Input: part model. Units: mm. Frame: model coordinates. Face numbers are marked on the shaded views. A direction names the side the tool comes from. Round coordinates to 2 decimals unless told otherwise and drop trailing zeros. Loops run counter-clockwise (first coordinate to the right, second up) from the corner with the lowest first, then second, coordinate; pieces in that order, holes last. Notation, with made-up numbers: (-38.75, 2.25) - (-1.75, 2.25) arc R24 ccw to (-1.75, 18.25) - close; hole circle Ø2 at (-16, 70.25). An arc over 180 degrees is marked (long way). Write each question's results on one line, items separated by ' | '.
from build123d import *

# Parameters (mm, degrees)
F0_R     = 4.1
F0_R_2   = 1.625
F1_DEPTH = 15


with BuildPart() as f1:
    # F0 (on Top) → F1 (new body)
    with BuildSketch(Plane.XY):
        with BuildLine():
            Line((19.449329, 20.047105), (-17.462153, 20.047105))
            ThreePointArc((-17.462153, 20.047105), (-21.400342, 15.5), (-17.462153, 10.952895))
            ThreePointArc((-17.462153, 10.952895), (-13.583628, 11.018037), (-9.926019, 12.30997))
            ThreePointArc((-9.926019, 12.30997), (-0.583426, 14.431472), (8.979468, 13.851907))
            ThreePointArc((8.979468, 13.851907), (9.394135, 9.361936), (8.242019, 5.002531))
            ThreePointArc((8.242019, 5.002531), (7.672541, 2.530704), (7.5, 0))
            ThreePointArc((7.5, 0), (9.673183, -5.326817), (15, -7.5))
            ThreePointArc((15, -7.5), (20.326817, -5.326817), (22.5, 0))
            ThreePointArc((22.5, 0), (22.327459, 2.530704), (21.757981, 5.002531))
            ThreePointArc((21.757981, 5.002531), (21.215093, 9.858766), (22.510411, 14.570442))
            ThreePointArc((22.510411, 14.570442), (22.434346, 18.121727), (19.449329, 20.047105))
        make_face()
        with Locations((15, 0)):
            Circle(F0_R, mode=Mode.SUBTRACT)
        with Locations((15.5, 15.5)):
            Circle(F0_R_2, mode=Mode.SUBTRACT)
    extrude(amount=F1_DEPTH)


solid = f1.part
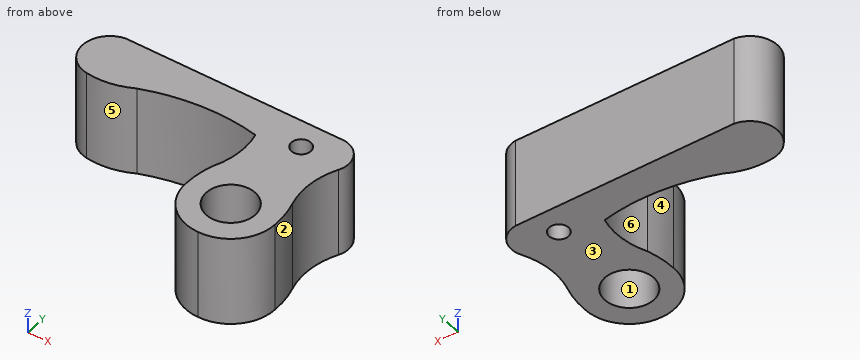
1. Line query: line 1 (Y direction, x = 15.5, z = 9) (3 decimals); line 2 (Y direction, x = 15, z = 12); line 3 (X direction, y = 15.75, z = 7.75). Output: solid intervals per line, ascending. Write a range as [from, to].
Answer:
line 1: [-7.488, -4.069], [4.069, 13.875], [17.125, 20.047] | line 2: [-7.5, -4.1], [4.1, 13.95], [17.05, 20.05] | line 3: [-21.39, 13.89], [17.11, 22.88]
2. Set-up query: the marked faces 1 and 2. Return all of +Z, -Z, +X, -X, +Y, -Y with unobstructed straight access to the full face (end or side cutting, diameter ignored); none if empty.
Answer:
face 1: +Z, -Z | face 2: +Z, -Z, +X
3. Section query D-D, the plane y = 15.5. Output: boundary loops of the cut face in (x, z) (1 decimal).
Answer:
outline: (-21.4, 0) - (13.9, 0) - (13.9, 15) - (-21.4, 15) - close; (17.1, 0) - (22.8, 0) - (22.8, 15) - (17.1, 15) - close
4. Contact query for flat-ended pins moving along their axis: pin 1 (3 mm diameter, centred on x = 12.5, z = 8, fed in from -Y); pin 2 (5 mm diameter, centred on y = 12.5, z = 11.5, fed in from +X); pin 3 (4 mm diameter, centred on x = 5, z = 6.5, fed in from -Y); pin 4 (13 mm diameter, centred on x = 15, y = 0, fed in from -Z). Output: stop coordinate, or through.
Answer:
pin 1: y = -7.44 | pin 2: x = 22.69 | pin 3: y = 14.2 | pin 4: z = 0
5. Section query B-B, the plane z = 14.25. Output: boundary loops of the cut face in (x, y) (3 decimals), plus the area to 3 significant figures.
Answer:
outline: (-17.462, 10.953) arc R12.071 ccw to (-9.926, 12.31) arc R33.868 cw to (8.979, 13.852) arc R12.932 cw to (8.242, 5.003) arc R16.034 ccw to (7.5, 0) arc R7.421 ccw to (15, -7.5) arc R7.421 ccw to (22.5, 0) arc R16.034 ccw to (21.758, 5.003) arc R12.95 cw to (22.51, 14.57) arc R3.786 ccw to (19.449, 20.047) - (-17.462, 20.047) arc R4.594 ccw to start; hole circle Ø8.2 at (15, 0); hole circle Ø3.25 at (15.5, 15.5) | area: 500 mm^2
6. Mould query, pull axis Y, two halves, no side actions, for the marked faces 3, 4, 5 and 6. Classes: pulls with the +Y half, pulls with the -Y half, needs draft (parallel to the pull), parting line crosses it, or undercut.
Answer:
face 3: needs draft | face 4: undercut | face 5: pulls with the -Y half | face 6: undercut
7. Section query A-A, the plane x = 16.5. Output: boundary loops of the cut face in (y, z), plus the area to 3 significant figures.
Answer:
outline: (-7.36, 0) - (-3.82, 0) - (-3.82, 15) - (-7.36, 15) - close; (3.82, 0) - (14.22, 0) - (14.22, 15) - (3.82, 15) - close; (16.78, 0) - (20.05, 0) - (20.05, 15) - (16.78, 15) - close | area: 258 mm^2
8. Section query C-C, the plane y = -2.25. Output: boundary loops of the cut face in (x, z).
Answer:
outline: (7.82, 0) - (11.57, 0) - (11.57, 15) - (7.82, 15) - close; (18.43, 0) - (22.18, 0) - (22.18, 15) - (18.43, 15) - close
